from build123d import *

# Parameters (mm, degrees)
ESBO_O1_W                  = 170
ESBO_O1_H                  = 30
RESSALTO_EXTRUS_O1_DEPTH   = 150
CORTE_EXTRUS_O1_DEPTH      = 222
CORTE_EXTRUS_O1_DEPTH_BACK = 36
RESSALTO_EXTRUS_O2_DEPTH   = 5
RESSALTO_EXTRUS_O3_DEPTH   = 5
ESBO_O4_W                  = 159.333333333
ESBO_O4_H                  = 140.588235294
CORTE_EXTRUS_O2_DEPTH      = 25
CORTE_EXTRUS_O3_DEPTH      = 31
CORTE_EXTRUS_O4_DEPTH      = 42
FILETE1_R                  = 10
CORTE_EXTRUS_O5_DEPTH      = 32
CORTE_EXTRUS_O6_START      = -15.72292277
CORTE_EXTRUS_O6_OUTLINE_R  = 3.95
CORTE_EXTRUS_O6_DEPTH      = 4.876648775
CORTE_EXTRUS_O7_START      = -132.751356438
CORTE_EXTRUS_O7_OUTLINE_R  = 3.95
CORTE_EXTRUS_O7_DEPTH      = 3.479370229
RESSALTO_EXTRUS_O6_DEPTH   = 17
RESSALTO_EXTRUS_O7_DEPTH   = 4
CORTE_EXTRUS_O8_DEPTH      = 21
F_3DSKETCH12_R             = 1.5
CORTE_EXTRUS_O9_DEPTH      = 14
CORTE_EXTRUS_O10_DEPTH     = 19
ESBO_O11_W                 = 17.407525744
ESBO_O11_H                 = 16.792397695
CORTE_EXTRUS_O11_DEPTH     = 10
CORTE_EXTRUS_O12_DEPTH     = 20
CORTE_EXTRUS_O13_DEPTH     = 14
ESBO_O12_W                 = 182.438351364
ESBO_O12_H                 = 161.616583002
CORTE_EXTRUS_O14_DEPTH     = 90


# Read off the part's stored shape, not the designer's step: Corte-extrusão6, Corte-extrusão7
with BuildPart() as part:
    # Esboço1 → Ressalto-extrusão1 (new body)
    with BuildSketch(Plane(origin=(0, 0, 0), x_dir=(1, 0, 0), z_dir=(0, 1, 0))):
        with Locations((85, 15)):
            Rectangle(ESBO_O1_W, ESBO_O1_H)
        Polygon((80, 160), (0, 30), (170, 30), (170, 160), align=None)
        Polygon((170, 160), (170, 185), (80, 160), align=None)
    extrude(amount=RESSALTO_EXTRUS_O1_DEPTH)

    # Esboço2 → Corte-extrusão1 (cut, two sides: drawn at the far end of the back side and taken through both)
    with BuildSketch(Plane(origin=(0, 0, 0), x_dir=(1, 0, 0), z_dir=(0, 1, 0)).offset(-CORTE_EXTRUS_O1_DEPTH_BACK)):
        Polygon((84.391050739, 157.608625205), (165, 180), (165, 5), (5, 5), (5, 29.866892941), align=None)
    extrude(amount=CORTE_EXTRUS_O1_DEPTH + CORTE_EXTRUS_O1_DEPTH_BACK, mode=Mode.SUBTRACT)

    # Esboço3 → Ressalto-extrusão2 (add)
    with BuildSketch(Plane(origin=(0, 0, 0), x_dir=(1, 0, 0), z_dir=(0, 1, 0))):
        Polygon((84.391050739, 157.608625205), (165, 180), (165, 5), (5, 5), (5, 29.866892941), align=None)
    extrude(amount=RESSALTO_EXTRUS_O2_DEPTH)

    # 3DSketch2 → Ressalto-extrusão3 (add)
    with BuildSketch(Plane(origin=(165, 150, -5), x_dir=(0, 0, -1), z_dir=(0, 1, 0))):
        Polygon((0, 0), (0, 160), (24.866892941, 160), (152.608625205, 80.608949261), (175, 0), align=None)
    extrude(amount=-RESSALTO_EXTRUS_O3_DEPTH)

    # Esboço4 → Corte-extrusão2 (cut)
    with BuildSketch(Plane.XY):
        with Locations((85.333333333, 74.705882353)):
            Rectangle(ESBO_O4_W, ESBO_O4_H)
    extrude(amount=-CORTE_EXTRUS_O2_DEPTH, mode=Mode.SUBTRACT)

    # 3DSketch3 → Corte-extrusão3 (cut)
    with BuildSketch(Plane(origin=(74.759025743, 90, -151.483416833), x_dir=(-0.29071694485714406, -0.8320502943378435, 0.4724150353928592), z_dir=(-0.8516583167045438, 0, -0.5240974256643346))):
        Polygon((0, 0), (22.188007849, 33.282011774), (72.111025509, 0), (49.92301766, -33.282011774), align=None)
    extrude(amount=-CORTE_EXTRUS_O3_DEPTH, mode=Mode.SUBTRACT)

    # 3DSketch4 → Corte-extrusão4 (cut)
    with BuildSketch(Plane(origin=(69.518051487, 130, -142.966833666), x_dir=(-0.37059284368967266, -0.7071067811865471, 0.6022133709956982), z_dir=(0.8516583167045362, 0, 0.5240974256643472))):
        Polygon((0, 0), (14.142135624, -14.142135624), (28.284271247, 0), (14.142135624, 14.142135624), align=None)
    extrude(amount=CORTE_EXTRUS_O4_DEPTH, mode=Mode.SUBTRACT)

    # Filete1
    filete1_edges = [part.edges().sort_by_distance(p)[0] for p in [
        (170, 75, -185),
        (125, 0, -172.5),
        (125, 150, -172.5),
        (80, 75, -160),
        (40, 0, -95),
        (40, 150, -95),
        (0, 75, -30),
        (84.391050739, 75, -157.608625205),
    ]]
    fillet(filete1_edges, radius=FILETE1_R)

    # 3DSketch5 → Corte-extrusão5 (cut)
    with BuildSketch(Plane(origin=(38.121221288, 25, -91.946984593), x_dir=(-0.194644897392922, 0.9284766908852593, 0.31629795826349816), z_dir=(0.851658316704544, 0, 0.5240974256643347))):
        Polygon((0, 0), (14.855627054, 37.139067635), (107.703296143, 0), (92.847669089, -37.139067635), align=None)
    extrude(amount=CORTE_EXTRUS_O5_DEPTH, mode=Mode.SUBTRACT)

    # Corte-extrusão6 outline → Corte-extrusão6 (cut)
    with BuildSketch(Plane(origin=(0, 0, 0), x_dir=(0.5240974256643349, 0, -0.8516583167045437), z_dir=(0.8516583167045437, 0, 0.5240974256643349)).offset(CORTE_EXTRUS_O6_START)):
        with Locations((148.193124726, 20)):
            Circle(CORTE_EXTRUS_O6_OUTLINE_R)
    extrude(amount=CORTE_EXTRUS_O6_DEPTH, mode=Mode.SUBTRACT)

    # Corte-extrusão7 outline → Corte-extrusão7 (cut)
    with BuildSketch(Plane(origin=(0, 0, 0), x_dir=(0.9635179096299408, 0, -0.267643863786094), z_dir=(0.267643863786094, 0, 0.9635179096299409)).offset(CORTE_EXTRUS_O7_START)):
        with Locations((161.993020775, 122.164347625)):
            Circle(CORTE_EXTRUS_O7_OUTLINE_R)
    extrude(amount=CORTE_EXTRUS_O7_DEPTH, mode=Mode.SUBTRACT)

    # 3DSketch9 → Ressalto-extrusão6 (add)
    with BuildSketch(Plane(origin=(76.350750718, 26, -154.069969916), x_dir=(-0.29815073011621673, 0.8224176546598938, 0.4844949364388514), z_dir=(0.8516583167045438, 0, 0.5240974256643349))):
        Polygon((0, 0), (26.758649409, 38.684123705), (82.683049926, 0), (55.924400517, -38.684123705), align=None)
        Polygon((5.017416454, 0.222210211), (27.772783339, 33.118916398), (77.117842619, -1.01413393), (54.362475733, -33.910840117), align=None, mode=Mode.SUBTRACT)
    extrude(amount=RESSALTO_EXTRUS_O6_DEPTH)

    # 3DSketch10 → Ressalto-extrusão7 (add, along a direction that is not the sketch's normal)
    with BuildSketch(Plane(origin=(0, 0, 0), x_dir=(0.7498378553650926, 0.6616216370868463, 0), z_dir=(0, 0, 1))):
        with BuildLine():
            Line((0, 0), (14.996757107, -13.232432742))
            Line((14.996757107, -13.232432742), (28.229189849, 1.764324366))
            ThreePointArc((28.229189849, 1.764324366), (21.556867541, 14.536675999), (25.141622209, 28.493838504))
            Line((25.141622209, 28.493838504), (13.232432742, 14.996757107))
            Line((13.232432742, 14.996757107), (0, 0))
        make_face()
        with BuildLine():
            Line((99.243245563, 112.475678305), (115.742930564, 97.917132715))
            Line((115.742930564, 97.917132715), (100.070543679, 80.155094246))
            ThreePointArc((100.070543679, 80.155094246), (86.055529464, 85.755516688), (71.66166921, 81.216558438))
            Line((71.66166921, 81.216558438), (83.570858678, 94.713639835))
            Line((83.570858678, 94.713639835), (99.243245563, 112.475678305))
        make_face()
        Polygon((226.715680975, 0), (211.718923868, 13.232432742), (198.486491126, -1.764324366), (213.483248233, -14.996757107), align=None)
        Polygon((127.472435412, -112.475678305), (112.475678305, -99.243245563), (125.708111047, -84.246488456), (140.704868154, -97.478921197), align=None)
    extrude(amount=-RESSALTO_EXTRUS_O7_DEPTH, dir=(0.26764386378609445, 0, 0.9635179096299407))

    # 3DSketch11 → Corte-extrusão8 (cut)
    with BuildSketch(Plane(origin=(153.100052242, 17.26943239, -180.305570067), x_dir=(-0.07376023038027929, 0.9970655099962036, 0.02048895288341091), z_dir=(0.2676438637860946, 0, 0.9635179096299407))):
        Polygon((0, 0), (0.269964353, 3.516152018), (46.066103253, 0), (45.7961389, -3.516152018), align=None)
    extrude(amount=CORTE_EXTRUS_O8_DEPTH, mode=Mode.SUBTRACT)

    # 3DSketch12 → Corte-extrusão9 (cut)
    with BuildSketch(Plane(origin=(160, 140, 0), x_dir=(-0.7560654573770964, -0.6544960077503622, 0), z_dir=(0, 0, 1))):
        with Locations(Location((0, 0, 0), (0, 0, 319.118554366))):
            Circle(F_3DSKETCH12_R)
        with Locations(Location((85.084481008, 98.288509459, 0), (0, 0, 319.118554366))):
            Circle(F_3DSKETCH12_R)
        with Locations(Location((113.858951537, -96.124361942, 0), (0, 0, 139.118554366))):
            Circle(F_3DSKETCH12_R)
        with Locations(Location((196.909602971, 0, 0), (0, 0, 139.118554366))):
            Circle(F_3DSKETCH12_R)
    extrude(amount=-CORTE_EXTRUS_O9_DEPTH, mode=Mode.SUBTRACT)

    # 3DSketch13 → Corte-extrusão10 (cut)
    with BuildSketch(Plane(origin=(170, 70.245878967, 0), x_dir=(0, -0.4354246522459521, -0.9002251786172678), z_dir=(-1, 0, 0))):
        Polygon((0, 0), (32.261446294, -15.604350297), (39.809023237, 0), (7.547576943, 15.604350297), align=None)
    extrude(amount=CORTE_EXTRUS_O10_DEPTH, mode=Mode.SUBTRACT)

    # Esboço11 → Corte-extrusão11 (cut)
    with BuildSketch(Plane(origin=(170, 0, 0), x_dir=(0, 0, -1), z_dir=(1, 0, 0))):
        with Locations((8.703762872, 30.096304842)):
            Rectangle(ESBO_O11_W, ESBO_O11_H)
    extrude(amount=-CORTE_EXTRUS_O11_DEPTH, mode=Mode.SUBTRACT)

    # 3DSketch14 → Corte-extrusão12 (cut)
    with BuildSketch(Plane(origin=(170, 87.396079578, 0), x_dir=(0, -0.09341146144778735, -0.9956275904524686), z_dir=(1, 0, 0))):
        Polygon((0, 0), (20.627912038, 1.935345533), (19.506160301, 13.891554783), (-1.121751737, 11.956209249), align=None)
        Polygon((-2.576084268, 27.457236328), (18.165947056, 29.403288726), (16.691971594, 45.113680317), (-4.050059731, 43.167627919), align=None)
        Polygon((91.534016736, 10.656116635), (99.096194716, 11.679615344), (100.676965661, 0), (93.114787682, -1.02349871), align=None)
    extrude(amount=-CORTE_EXTRUS_O12_DEPTH, mode=Mode.SUBTRACT)

    # 3DSketch15 → Corte-extrusão13 (cut)
    with BuildSketch(Plane(origin=(129.748977416, 150, 0), x_dir=(-0.6170578351280018, 0, -0.7869178026370631), z_dir=(0, -1, 0))):
        Polygon((0, 0), (11.819817446, 9.268453377), (19.087630878, 0), (7.267813432, -9.268453377), align=None)
    extrude(amount=CORTE_EXTRUS_O13_DEPTH, mode=Mode.SUBTRACT)

    # Esboço12 → Corte-extrusão14 (cut)
    with BuildSketch(Plane.XY):
        with Locations((84.195107922, 72.896320561)):
            Rectangle(ESBO_O12_W, ESBO_O12_H)
    extrude(amount=-CORTE_EXTRUS_O14_DEPTH, mode=Mode.SUBTRACT)


solid = part.part
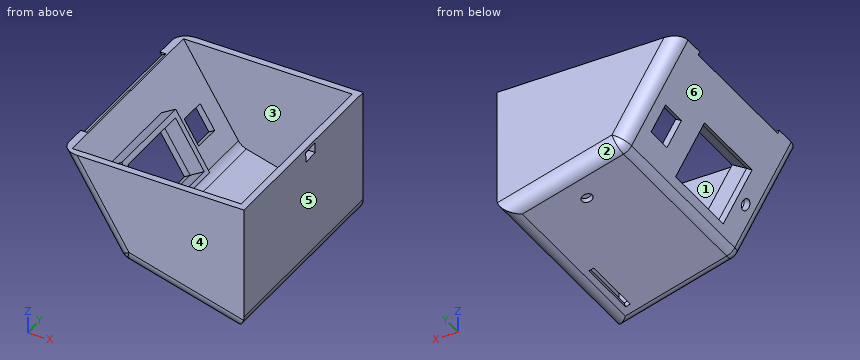
Work out the finished part from the listing and answer in its coordinate system (mm). Face numbers are marked on the shaded views. A direction names the side the tool comes from. Round coordinates to 2 decimals unless told otherwise and drop trailing zeros. Loops run counter-clockwise (first coordinate to the right, second up) from the corner with the lowest first, then second, coordinate; pieces in that order, holes last. Notation, with made-up numbers: (63.5, 15) -> (70.5, 15) arc R19 ccw to (70.5, 36) -> close; hole circle Ø3 at (16, 16). An arc over 180 degrees is marked (long way). Use one line per item in the form item = value.
(1) Find section A-A on y = 41.5. Give the vertices of the cut face in (x, z).
Answer list:
outline = (38.12, -91.95) -> (53.8, -117.42) -> (68.27, -108.51) -> (66.18, -105.1) -> (55.75, -111.52) -> (42.37, -90) -> (41.29, -90) -> close; (74.76, -151.48) -> (77.94, -156.66) arc R10 ccw to (83.78, -161.05) -> (149.7, -179.36) -> (150.63, -176.01) -> (88.15, -158.65) arc R10 cw to (82.33, -154.3) -> (80.58, -151.47) -> (90.83, -145.16) -> (89.24, -142.57) -> close; (153.1, -180.31) -> (157.32, -181.48) arc R10 ccw to (170, -171.84) -> (170, -90) -> (165, -90) -> (165, -180) -> (154.03, -176.95) -> close
(2) Flat-ended cylindrical pins translate along their axes: P1, Ø4.5, axis at x = 152.5, z = -177.5, coming from the -Y side; P2, Ø12, axis at x = 71.5, y = 38.5, coming from the +Z side; P3, Ø2, axis at x = 151, z = -178.5, coming from the +Y side. Find the tip coordinate at first contact, or state that the pin passes through.
Answer list:
P1 = 1.46
P2 = -105.1
P3 = 146.23
(3) A tool of negligible diameter and unlimited length cuts with its end or side. For the marked faces 1 and 2, from which of +Z, -Z, +X, -X, +Y, -Y can it reach the whole face along a straight path? Write none if from no direction.
Answer list:
face_1 = +Z
face_2 = -Z, -X, +Y
(4) Find section C-C on z = -132. Give the number of separate pieces and of enclosed holes in the cut face, then the cut area to 3 significant figures.
Answer list:
separate_pieces = 3
enclosed_holes = 0
area = 2,140 mm2
(5) For a pull along X with two mould halves and no side action, classify the marked faces 3, 4, 5 and 6 as released by +X, released by -X, zero draft, split by the parting line, or undercut.
Answer list:
face_3 = undercut
face_4 = zero draft
face_5 = released by +X
face_6 = released by -X
(6) Find section B-B on y = 69.5. Give the vertices of the cut face in (x, z), then the cut area to 3 significant figures.
Answer list:
outline = (38.12, -91.95) -> (53.8, -117.42) -> (68.27, -108.51) -> (66.18, -105.1) -> (55.75, -111.52) -> (42.37, -90) -> (41.29, -90) -> close; (74.76, -151.48) -> (77.94, -156.66) arc R10 ccw to (83.78, -161.05) -> (157.32, -181.48) arc R10 ccw to (170, -171.84) -> (170, -90) -> (165, -90) -> (165, -180) -> (88.15, -158.65) arc R10 cw to (82.33, -154.3) -> (80.58, -151.47) -> (90.83, -145.16) -> (89.24, -142.57) -> close
area = 1,010 mm2
(7) Straight lines are drawn through the part: line 1 (Y direction, x = 157, z = -112); line 2 (X direction, y = 116, z = -151.5); line 3 (X direction, y = 96.5, z = -112.5). For each, find the intervals that lie inside material, in ascending order.
Answer list:
line_1 = 0 to 5, 145 to 150
line_2 = 74.77 to 80.59, 165 to 170
line_3 = 50.77 to 56.36, 165 to 170
